Geometry: final body of the model. Coordinates: model frame, mm. Face numbers are marked on the shaded views. A direction names the side the tool comes from. Give positions to 0.01 mm unless a question says otherwise; leave off trailing zeros. Loops run counter-clockwise (first coordinate to the right, second up) from the corner with the lowest first, then second, coordinate; pieces in that order, holes last. Notation, with made-up numbers: (65, -35) -> (85, -35) arc R28 ccw to (85, 0) -> close; hole circle Ø3 at (-1, 69.5). An arc over 180 degrees is marked (long way). Answer in a Markdown table with one row per item. Add a question column.
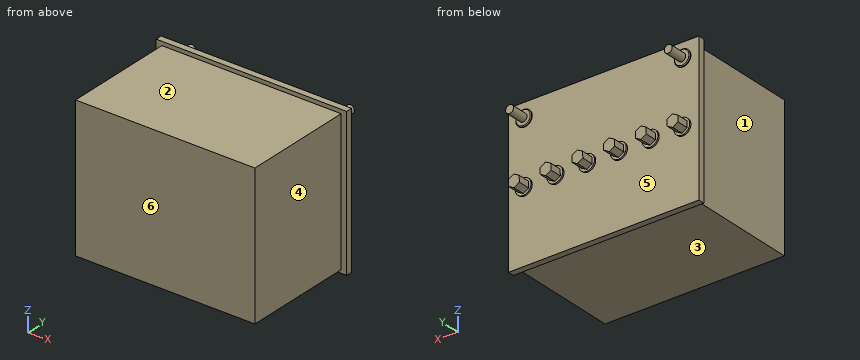
from build123d import *

# Parameters (mm, degrees)
SKETCH2_W           = 113
SKETCH2_H           = 70
BOSS_EXTRUDE2_DEPTH = 89
SKETCH3_W           = 120
SKETCH3_H           = 93.6
BOSS_EXTRUDE3_DEPTH = 4
SKETCH5_R           = 5
BOSS_EXTRUDE4_DEPTH = 1
BOSS_EXTRUDE5_DEPTH = 7.5
SKETCH9_R           = 5
BOSS_EXTRUDE6_DEPTH = 1
SKETCH11_R          = 2.5
BOSS_EXTRUDE7_DEPTH = 11


with BuildPart() as part:
    # Sketch2 → Boss-Extrude2 (new body)
    with BuildSketch(Plane.XY):
        with Locations((56.5, -35)):
            Rectangle(SKETCH2_W, SKETCH2_H)
    extrude(amount=BOSS_EXTRUDE2_DEPTH)

    # Sketch3 → Boss-Extrude3 (add)
    with BuildSketch(Plane(origin=(0, 0, 0), x_dir=(1, 0, 0), z_dir=(0, 1, 0))):
        with Locations((56.443629761, -44.692561868)):
            Rectangle(SKETCH3_W, SKETCH3_H)
    extrude(amount=BOSS_EXTRUDE3_DEPTH)

    # Sketch5 → Boss-Extrude4 (add)
    with BuildSketch(Plane(origin=(0, 4, 0), x_dir=(1, 0, 0), z_dir=(0, 1, 0))):
        with Locations(Location((6.443629761, -42.892561868, 0), (0, 0, 270))):
            Circle(SKETCH5_R)
        with Locations(Location((26.443629761, -42.892561868, 0), (0, 0, 270))):
            Circle(SKETCH5_R)
        with Locations(Location((46.443629761, -42.892561868, 0), (0, 0, 270))):
            Circle(SKETCH5_R)
        with Locations(Location((66.443629761, -42.892561868, 0), (0, 0, 270))):
            Circle(SKETCH5_R)
        with Locations(Location((86.443629761, -42.892561868, 0), (0, 0, 270))):
            Circle(SKETCH5_R)
        with Locations(Location((106.443629761, -42.892561868, 0), (0, 0, 270))):
            Circle(SKETCH5_R)
    extrude(amount=BOSS_EXTRUDE4_DEPTH)

    # Sketch7 → Boss-Extrude5 (add)
    with BuildSketch(Plane(origin=(0, 5, 0), x_dir=(1, 0, 0), z_dir=(0, 1, 0))):
        Polygon((29.878505301, -44.792186338), (29.80619058, -40.867684626), (26.37131504, -38.968060156), (23.008754221, -40.992937397), (23.081068941, -44.917439109), (26.515944482, -46.81706358), align=None)
        Polygon((9.878505301, -44.792186338), (9.80619058, -40.867684626), (6.37131504, -38.968060156), (3.008754221, -40.992937397), (3.081068941, -44.917439109), (6.515944482, -46.81706358), align=None)
        Polygon((49.878505301, -44.792186338), (49.80619058, -40.867684626), (46.37131504, -38.968060156), (43.008754221, -40.992937397), (43.081068941, -44.917439109), (46.515944482, -46.81706358), align=None)
        Polygon((69.878505301, -44.792186338), (69.80619058, -40.867684626), (66.37131504, -38.968060156), (63.008754221, -40.992937397), (63.081068941, -44.917439109), (66.515944482, -46.81706358), align=None)
        Polygon((89.878505301, -44.792186338), (89.80619058, -40.867684626), (86.37131504, -38.968060156), (83.008754221, -40.992937397), (83.081068941, -44.917439109), (86.515944482, -46.81706358), align=None)
        Polygon((109.878505301, -44.792186338), (109.80619058, -40.867684626), (106.37131504, -38.968060156), (103.008754221, -40.992937397), (103.081068941, -44.917439109), (106.515944482, -46.81706358), align=None)
    extrude(amount=BOSS_EXTRUDE5_DEPTH)

    # Sketch9 → Boss-Extrude6 (add)
    with BuildSketch(Plane(origin=(0, 4, 0), x_dir=(1, 0, 0), z_dir=(0, 1, 0))):
        with Locations(Location((6.443629761, -82.263237169, 0), (0, 0, 270))):
            Circle(SKETCH9_R)
        with Locations(Location((106.443629761, -82.263237169, 0), (0, 0, 270))):
            Circle(SKETCH9_R)
    extrude(amount=BOSS_EXTRUDE6_DEPTH)

    # Fillet5: read off the stored shape, not the designer's step
    # Fillet5 outline → Fillet5 (revolve, cut)
    with BuildSketch(Plane(origin=(6.443629761, 0, 82.263237169), x_dir=(1, 0, 0), z_dir=(0, 0, 1))):
        Polygon((5, 5), (4.5, 5), (5, 4.5), align=None)
    revolve(axis=Axis((6.443629761, 0, 82.263237169), (0, 1, 0)), mode=Mode.SUBTRACT)

    # Fillet7: read off the stored shape, not the designer's step
    # Fillet7 outline → Fillet7 (revolve, cut)
    with BuildSketch(Plane(origin=(106.443629761, 0, 82.263237169), x_dir=(1, 0, 0), z_dir=(0, 0, 1))):
        Polygon((5, 5), (4.5, 5), (5, 4.5), align=None)
    revolve(axis=Axis((106.443629761, 0, 82.263237169), (0, 1, 0)), mode=Mode.SUBTRACT)

    # Sketch11 → Boss-Extrude7 (add)
    with BuildSketch(Plane(origin=(0, 5, 0), x_dir=(1, 0, 0), z_dir=(0, 1, 0))):
        with Locations(Location((6.443629761, -82.263237169, 0), (0, 0, 270))):
            Circle(SKETCH11_R)
        with Locations(Location((106.443629761, -82.263237169, 0), (0, 0, 270))):
            Circle(SKETCH11_R)
    extrude(amount=BOSS_EXTRUDE7_DEPTH)


solid = part.part
(1) Material intervals for line 1 along Y through (x, z) = (75, 64.5); line 2 along X through (y, z) = (-60, 52); line 3 along Z through (x, y) = (75, -36.5), sorted ascending. Write a range as from..to.
(2) Cut plane A-A on z = 74.5. Return the cut outline in (x, y).
(3) Draft query along X for the marked faces 4, 5 and 6. Return one class per face: +X half, -X half, draft (parallel to the pull), parting line (faces both ways), or undercut.
(4) Cut plane B-B on x = 53.5. Return the cut outline in (y, z), then the cut area to 3 significant figures.
(5) Cut plane C-C on y = -29. Return the cut outline in (x, z).
(6) Pin query (flat end, axial travel): pin 1 Ø6 at (y, z) = (-19.5, 70) entering from +X; pin 2 Ø3 at (x, z) = (18.5, 12.5) entering from +Y; pin 3 Ø1 at (y, z) = (-30.5, 80) entering from -X. Return the tip coordinate at first contact, or that it passes through.
(7) Reachability of the marked faces 1, 2 and 3 from +Z, -Z, +X, -X, +Y, -Y: full face, straight path, thin tool, end or side. Return the list, or none.
Answer list:
| question | item | result |
|---|---|---|
| 1 | line 1 | y = -70..4 |
| 1 | line 2 | x = 0..113 |
| 1 | line 3 | z = 0..89 |
| 2 | outline | (-3.56, 0) -> (0, 0) -> (0, -70) -> (113, -70) -> (113, 0) -> (116.44, 0) -> (116.44, 4) -> (-3.56, 4) -> close |
| 3 | face 4 | +X half |
| 3 | face 5 | undercut |
| 3 | face 6 | draft |
| 4 | outline | (-70, 0) -> (0, 0) -> (0, -2.11) -> (4, -2.11) -> (4, 91.49) -> (0, 91.49) -> (0, 89) -> (-70, 89) -> close |
| 4 | area | 6,600 mm² |
| 5 | outline | (0, 0) -> (113, 0) -> (113, 89) -> (0, 89) -> close |
| 6 | pin 1 | stops at x = 113 |
| 6 | pin 2 | stops at y = 4 |
| 6 | pin 3 | stops at x = 0 |
| 7 | face 1 | +Z, -Z, -X, -Y |
| 7 | face 2 | +Z, +X, -X, -Y |
| 7 | face 3 | -Z, +X, -X, -Y |
